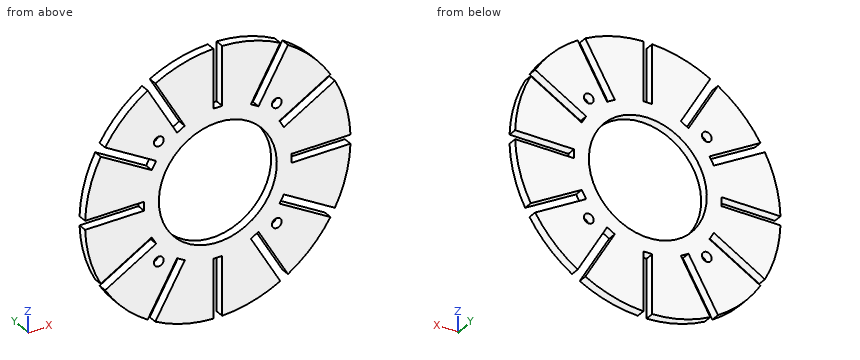
from build123d import *

# Parameters (mm, degrees)
SKETCH1_R           = 45
SKETCH1_R_2         = 10
BOSS_EXTRUDE1_DEPTH = 1.5
SKETCH2_R           = 1.65
CUT_EXTRUDE1_DEPTH  = 10
SKETCH3_W           = 3
SKETCH3_H           = 20
SKETCH3_W_2         = 20
SKETCH3_H_2         = 3
CUT_EXTRUDE2_DEPTH  = 10
SKETCH4_R           = 20
CUT_EXTRUDE3_DEPTH  = 10


with BuildPart() as part:
    # Sketch1 → Boss-Extrude1 (new, symmetric)
    with BuildSketch(Plane(origin=(0, 0, 0), x_dir=(1, 0, 0), z_dir=(0, 1, 0))):
        with Locations(Location((0, 0, 0), (0, 0, 270))):
            Circle(SKETCH1_R)
        with Locations(Location((0, 0, 0), (0, 0, 270))):
            Circle(SKETCH1_R_2, mode=Mode.SUBTRACT)
    extrude(amount=BOSS_EXTRUDE1_DEPTH, both=True)

    # Sketch2 → Cut-Extrude1 (cut)
    with BuildSketch(Plane(origin=(0, 1.5, 0), x_dir=(1, 0, 0), z_dir=(0, 1, 0))):
        with Locations(Location((-20, -20, 0), (0, 0, 270))):
            Circle(SKETCH2_R)
        with Locations(Location((-20, 20, 0), (0, 0, 270))):
            Circle(SKETCH2_R)
        with Locations(Location((20, 20, 0), (0, 0, 270))):
            Circle(SKETCH2_R)
        with Locations(Location((20, -20, 0), (0, 0, 270))):
            Circle(SKETCH2_R)
    extrude(amount=-CUT_EXTRUDE1_DEPTH, mode=Mode.SUBTRACT)

    # Sketch3 → Cut-Extrude2 (cut)
    with BuildSketch(Plane(origin=(0, 1.5, 0), x_dir=(1, 0, 0), z_dir=(0, 1, 0))):
        with Locations((0, -35)):
            Rectangle(SKETCH3_W, SKETCH3_H)
        Polygon((-13.799038106, -20.900635095), (-23.799038106, -38.22114317), (-21.200961894, -39.72114317), (-11.200961894, -22.400635095), align=None)
        Polygon((-22.400635095, -11.200961894), (-39.72114317, -21.200961894), (-38.22114317, -23.799038106), (-20.900635095, -13.799038106), align=None)
        with Locations((-35, 0)):
            Rectangle(SKETCH3_W_2, SKETCH3_H_2)
        Polygon((-20.900635095, 13.799038106), (-38.22114317, 23.799038106), (-39.72114317, 21.200961894), (-22.400635095, 11.200961894), align=None)
        Polygon((-11.200961894, 22.400635095), (-21.200961894, 39.72114317), (-23.799038106, 38.22114317), (-13.799038106, 20.900635095), align=None)
        with Locations((0, 35)):
            Rectangle(SKETCH3_W, SKETCH3_H)
        Polygon((13.799038106, 20.900635095), (23.799038106, 38.22114317), (21.200961894, 39.72114317), (11.200961894, 22.400635095), align=None)
        Polygon((22.400635095, 11.200961894), (39.72114317, 21.200961894), (38.22114317, 23.799038106), (20.900635095, 13.799038106), align=None)
        with Locations((35, 0)):
            Rectangle(SKETCH3_W_2, SKETCH3_H_2)
        Polygon((20.900635095, -13.799038106), (38.22114317, -23.799038106), (39.72114317, -21.200961894), (22.400635095, -11.200961894), align=None)
        Polygon((11.200961894, -22.400635095), (21.200961894, -39.72114317), (23.799038106, -38.22114317), (13.799038106, -20.900635095), align=None)
    extrude(amount=-CUT_EXTRUDE2_DEPTH, mode=Mode.SUBTRACT)

    # Sketch4 → Cut-Extrude3 (cut)
    with BuildSketch(Plane(origin=(0, 1.5, 0), x_dir=(1, 0, 0), z_dir=(0, 1, 0))):
        with Locations(Location((0, 0, 0), (0, 0, 270))):
            Circle(SKETCH4_R)
    extrude(amount=-CUT_EXTRUDE3_DEPTH, mode=Mode.SUBTRACT)


solid = part.part
Here's how the part is built. I have some questions about the finished solid (model axes, mm). Coordinates: 2 decimals unless noted, no trailing zeros. Order: outer loops, then holes, each group sorted by start corner. A loop starts at its lowest first (then second) coordinate and runs counter-clockwise, first axis right, second up. Notation, with made-up numbers: (57, 61) -> (91, 61) arc R5 ccw to (91, 70) -> close; hole circle Ø9 at (78, 53). An arc over 180 degrees is marked (long way). Answer in a Markdown table with one row per item.
(1) I want a section at A-A on x = 16. List the corners of the cut face in (y, z) for me, then the cut area to 3 significant figures.
Answer key:
| item | result |
|---|---|
| outline | (-1.5, -42.06) -> (1.5, -42.06) -> (1.5, -30.71) -> (-1.5, -30.71) -> close; (-1.5, -24.71) -> (1.5, -24.71) -> (1.5, -12) -> (-1.5, -12) -> close; (-1.5, 12) -> (1.5, 12) -> (1.5, 24.71) -> (-1.5, 24.71) -> close; (-1.5, 30.71) -> (1.5, 30.71) -> (1.5, 42.06) -> (-1.5, 42.06) -> close |
| area | 144 mm^2 |
(2) I want a section at D-D on y = 0.7. Count the separate pieces of the cut face and the enclosed holes in it, then the cut area to 3 significant figures.
Answer key:
| item | result |
|---|---|
| separate pieces | 1 |
| enclosed holes | 5 |
| area | 4,350 mm^2 |
(3) Please list where these lines run through material, in increasing order: probe 1 along Z at (x, y) = (18, 0); probe 2 along Z at (x, y) = (31, 1.35); probe 3 along X at (y, z) = (-0.95, 17.5).
Answer key:
| item | result |
|---|---|
| probe 1 | -41.24 to -34.18, -28.18 to -8.72, 8.72 to 28.18, 34.18 to 41.24 |
| probe 2 | -32.62 to -19.63, -16.17 to -1.5, 1.5 to 16.17, 19.63 to 32.62 |
| probe 3 | -41.46 to -33.31, -27.31 to -9.68, 9.68 to 27.31, 33.31 to 41.46 |
(4) Will these pins go through, and if not, where does the flat tip stop? pin 1 Ø1.5 at (x, y) = (-32.5, -0.5) entering from -Z; pin 2 Ø1.5 at (x, y) = (-39, -0.5) entering from +Z; pin 3 Ø1.5 at (y, z) = (0, 0.5) entering from -X.
Answer key:
| item | result |
|---|---|
| pin 1 | z = -31.89 |
| pin 2 | z = 21.19 |
| pin 3 | x = -25 |
(5) I want a section at B-B on z = 34.5. List the corners of the cut face in (x, y) for me, then the cut area to 3 significant figures.
Answer key:
| item | result |
|---|---|
| outline | (-28.89, -1.5) -> (-21.65, -1.5) -> (-21.65, 1.5) -> (-28.89, 1.5) -> close; (-18.19, -1.5) -> (-1.5, -1.5) -> (-1.5, 1.5) -> (-18.19, 1.5) -> close; (1.5, -1.5) -> (18.19, -1.5) -> (18.19, 1.5) -> (1.5, 1.5) -> close; (21.65, -1.5) -> (28.89, -1.5) -> (28.89, 1.5) -> (21.65, 1.5) -> close |
| area | 144 mm^2 |
(6) I want a section at C-C on x = 3. List the corners of the cut face in (y, z) for me, then the cut area to 3 significant figures.
Answer key:
| item | result |
|---|---|
| outline | (-1.5, -44.9) -> (1.5, -44.9) -> (1.5, -19.77) -> (-1.5, -19.77) -> close; (-1.5, 19.77) -> (1.5, 19.77) -> (1.5, 44.9) -> (-1.5, 44.9) -> close |
| area | 151 mm^2 |
